Read the model definition and answer for the solid it produces. Units are mm, in the model's axes. A direction names the side the tool comes from. Round coordinates to 2 decimals unless told otherwise and drop trailing zeros. Order: outer loops, then holes, each group sorted by start corner. A loop starts at its lowest first (then second) coordinate and runs counter-clockwise, first axis right, second up. Notation, with made-up numbers: M 34,33 L 83,33 A28 ccw 83,52 Z; hole C -8.75,-24.75 d4. An arc over 180 degrees is marked long. Use one line per item in the form item = value. Start each with the question number.
from build123d import *

# Parameters (mm, degrees)
PAD_DEPTH = 4


with BuildPart() as part:
    # Sketch → Pad (new body)
    with BuildSketch(Plane.XY):
        with BuildLine():
            Line((-10.75805, 41.603632), (-6, 41.603632))
            Line((-6, 41.603632), (-6, 16.603632))
            Line((-6, 16.603632), (6, 16.603632))
            Line((6, 16.603632), (6, 41.603632))
            Line((6, 41.603632), (10.75805, 41.603632))
            ThreePointArc((13.675637, 38.686046), (12.821096, 40.749091), (10.75805, 41.603632))
            Line((13.675637, 38.686046), (13.675637, 8.753459))
            Line((13.675637, 8.753459), (41.072293, -10.429886))
            ThreePointArc((41.659537, -13.76031), (42.055668, -11.973476), (41.072293, -10.429886))
            Line((41.659537, -13.76031), (37.519892, -19.672335))
            Line((37.519892, -19.672335), (17.041091, -5.332924))
            Line((17.041091, -5.332924), (4.422409, -23.354269))
            Line((4.422409, -23.354269), (46.213473, -47.482351))
            Line((46.213473, -47.482351), (43.278864, -52.565244))
            ThreePointArc((39.681503, -53.529154), (41.679816, -53.792237), (43.278864, -52.565244))
            Line((39.681503, -53.529154), (-7.047129, -26.550365))
            ThreePointArc((-12.952081, -16.322689), (-11.369854, -22.227641), (-7.047129, -26.550365))
            Line((-12.952081, -16.322689), (-12.952081, 39.409602))
            ThreePointArc((-10.75805, 41.603632), (-12.309464, 40.961015), (-12.952081, 39.409602))
        make_face()
    extrude(amount=PAD_DEPTH)


solid = part.part
Item 1: Section B-B (z = 2.6) is taken. Write down the section's boundary in (x, y), and give its area (3 significant figures).
Item 2: Section A-A (y = 35) is taken. Write down the section's boundary in (x, z), and give its area (3 significant figures).
Item 3: A tool of negligible diameter and unlimited length cuts with its end or side. For faces 1 (the flat face through (-6, 29, 2)), 2 (the flat face through (39.6, -16.7, 2)), 3 (the flat face through (27.42, -12.6, 1.97)), 4 (the cylindrical face through (-11.413, -22.153, 1.972)), from which of +Z, -Z, +X, -X, +Y, -Y can it reach the whole face along a straight path? Write none if from no direction.
Item 4: Given P1, Ø1, axis at x = 29.5, z = 3.5, coming from the -Y side; P2, Ø2, axis at y = -43, z = 2.5, coming from the -X side; P3, Ø2, axis at x = 17, z = 1.5, coming from the -Y side, each flat-ended and moving along its own axis, determine where each tip first touches the part or whether it passes through.
Item 5: Section D-D (y = 14) is taken. Write down the section's boundary in (x, z).
Item 6: Section C-C (x = 15) is taken. Write down the section's boundary in (y, z).
Item 7: For a pull along X with two mould halves and no side action, classify faces 5 (the flat face through (10, -5, 4)), 6 (the flat face through (27.18, -0.7, 1.97)), 7 (the flat face through (6, 29, 2)) as pulls with the +X half, pulls with the -X half, needs draft (parallel to the pull), parting line crosses it, or undercut.
Item 8: Find the intervals of material crossed by L1, parallel to X at y = 19, z = 2.75; L2, parallel to X at y = 13, z = 3.3; L3, parallel to X at y = -7, z = 1.85, in increasing order. Write a range as [from, to].
The answers:
q1.outline = M -12.95,-16.32 A11.81 ccw -7.05,-26.55 L 39.68,-53.53 A2.63 ccw 43.28,-52.57 L 46.21,-47.48 L 4.42,-23.35 L 17.04,-5.33 L 37.52,-19.67 L 41.66,-13.76 A2.39 ccw 41.07,-10.43 L 13.68,8.75 L 13.68,38.69 A2.92 ccw 10.76,41.6 L 6,41.6 L 6,16.6 L -6,16.6 L -6,41.6 L -10.76,41.6 A2.19 ccw -12.95,39.41 Z
q1.area = 2,150 mm²
q2.outline = M -12.95,0 L -6,0 L -6,4 L -12.95,4 Z; M 6,0 L 13.68,0 L 13.68,4 L 6,4 Z
q2.area = 58.5 mm²
q3.face_1 = +Z, -Z, +Y
q3.face_2 = +Z, -Z, +X
q3.face_3 = +Z, -Z
q3.face_4 = +Z, -Z, -X, -Y
q4.P1 = -47.94
q4.P2 = 19.71
q4.P3 = -41.01
q5.outline = M -12.95,0 L 13.68,0 L 13.68,4 L -12.95,4 Z
q6.outline = M -39.28,0 L -29.46,0 L -29.46,4 L -39.28,4 Z; M -8.25,0 L 7.83,0 L 7.83,4 L -8.25,4 Z
q7.face_5 = needs draft
q7.face_6 = pulls with the +X half
q7.face_7 = undercut
q8.L1 = [-12.95, -6], [6, 13.68]
q8.L2 = [-12.95, 13.68]
q8.L3 = [-12.95, 15.87], [19.42, 36.17]
